Can you work these out from the model? Positions are in its coordinate system, mm. A direction names the side the tool comes from. Coordinates: 2 decimals unless noted, no trailing zeros. Write each loop counter-clockwise with the first axis right and the second up, starting at its lowest first coordinate (ties: lowest second). Pieces come first, ordered by that corner, then holes. Notation, with made-up numbers: (51, 58.25) -> (102, 58.25) arc R18 cw to (102, 84.25) -> close; hole circle Ø4 at (9, 0). An arc over 180 degrees is marked (long way). Use one line per item in the form item = value.
Autodesk Inventor part; units mm, degrees
ref_plane "Work Plane1" through (0, 20, -19.05) normal (-1, 0, 0) x (0, 0, 1)
ref_plane "Work Plane2" through (6.5, 7, 0) normal (0, 0, -1) x (-1, 0, 0)
ref_plane "YZ Plane" through (0, 0, 0) normal (1, 0, 0) x (0, 1, 0)
sketch "Sketch1" plane through (0, 0, 0) normal (0, 1, 0) x (-1, 0, 0)
  line L0 (17.5, 19.05) -> (-17.5, 19.05)
  line L1 (-17.5, 19.05) -> (-17.5, -19.05)
  line L2 (-17.5, -19.05) -> (17.5, -19.05)
  line L3 (17.5, -19.05) -> (17.5, 19.05)
  line L4 (17.5, 19.05) -> (-17.5, -19.05) construction
  line L5 (-17.5, 19.05) -> (17.5, -19.05) construction
  point P0 (0, 0)
  dimension "d0" = 38.1
  dimension "d1" = 35
extrude "Extrusion1" add sketch "Sketch1" along normal blind 20
shell "Shell1" thickness 2 removed faces 1 at (5.8333, 20, -6.35)
sketch "Sketch2" plane through (-15.5, 2, 17.05) normal (0, 1, 0) x (1, 0, 0)
  line L0 (31, 34.1) -> (0, 34.1)
  line L1 (31, 0) -> (31, 34.1)
  line L2 (0, 34.1) -> (31, 34.1)
  line L3 (31, 34.1) -> (31, 0)
  line L4 (31, 0) -> (0, 0)
  line L5 (0, 0) -> (0, 34.1)
  point P0 (15.5, 17.05)
extrude "Extrusion2" add sketch "Sketch2" along normal blind 15.5
sketch "Sketch3" plane through (0, 20, 0) normal (0, 1, 0) x (1, 0, 0)
  line L0 (17.5, 19.05) -> (-17.5, 19.05)
  line L1 (-17.5, -19.05) -> (17.5, -19.05)
  line L2 (0, 19.05) -> (-6.5, 19.05)
  line L3 (-6.5, 19.05) -> (-6.5, -19.05)
  line L4 (-6.5, -19.05) -> (0, -19.05)
  line L5 (0, -19.05) -> (0, 19.05)
  point P0 (0, 0)
  dimension "d7" = 6.5
extrude "Extrusion3" cut sketch "Sketch3" against normal blind 13
ref_plane "Work Plane1" through (0, 20, -19.05) normal (-1, 0, 0) x (0, 0, 1)
mirror "Mirror1" about plane through (0, 20, -19.05) normal (-1, 0, 0) of "Extrusion3"
sketch "Sketch4" plane through (-15.5, 17.5, 17.05) normal (0, 1, 0) x (1, 0, 0)
  line L0 (22, -2) -> (22, 36.1)
  line L1 (22, 17.05) -> (26, 17.05)
  line L2 (26, 17.05) -> (26, 29.55)
  line L3 (26, 29.55) -> (22, 29.55)
  line L4 (22, 29.55) -> (22, 17.05)
  point P0 (15.5, 17.05)
  dimension "d11" = 4
  dimension "d12" = 12.5
extrude "Extrusion4" cut sketch "Sketch4" against normal up to surface (10.5 mm away)
sketch "Sketch5" plane through (-15.5, 17.5, 17.05) normal (0, 1, 0) x (1, 0, 0)
  line L0 (26, 17.05) -> (26, 29.55)
  line L1 (26, 17.05) -> (28.5, 17.05)
  line L2 (28.5, 17.05) -> (28.5, 26.85)
  line L3 (28.5, 26.85) -> (26, 26.85)
  line L4 (26, 26.85) -> (26, 17.05)
  point P0 (15.5, 17.05)
  dimension "d15" = 9.8
  dimension "d16" = 2.5
extrude "Extrusion5" cut sketch "Sketch5" against normal blind 12.7
sketch "Sketch6" plane through (0, 20, 0) normal (0, 1, 0) x (1, 0, 0)
  line L0 (15.5, 17.05) -> (15.5, -17.05)
  line L1 (15.5, 0) -> (19.9746, 0)
  line L2 (19.9746, 0) -> (19.9746, 7.5)
  line L3 (19.9746, 7.5) -> (15.5, 7.5)
  line L4 (15.5, 7.5) -> (15.5, 0)
  point P0 (0, 0)
  dimension "d19" = 7.5
extrude "Extrusion6" cut sketch "Sketch6" against normal up to surface (2.5 mm away)
ref_plane "Work Plane2" through (6.5, 7, 0) normal (0, 0, -1) x (-1, 0, 0)
mirror "Mirror2" about plane through (6.5, 7, 0) normal (0, 0, -1) of "Extrusion4", "Extrusion5", "Extrusion6"
sketch "Sketch7" plane through (-17.5, 0, -19.05) normal (-1, 0, 0) x (0, 0, 1)
  circle A0 centre (19.05, 12.14) radius 2.6
  line L0 (0, 20) -> (38.1, 20)
  point P0 (19.05, 0)
  dimension "d23" = 5.2
  dimension "d24" = 7.86
extrude "Extrusion7" cut sketch "Sketch7" against normal up to surface (11 mm away)
sketch "Sketch8" plane through (-17.5, 0, -19.05) normal (-1, 0, 0) x (0, 0, 1)
  circle A0 centre (19.05, 12.14) radius 2.6
  circle A1 centre (19.05, 12.14) radius 3.2
  point P0 (19.05, 0)
  dimension "d27" = 6.4
extrude "Extrusion8" cut sketch "Sketch8" against normal blind 9.5
fillet "Fillet1" radius 2 8 edges at (15.5, 18.75, -17.05) (-15.5, 18.75, -17.05) (-15.5, 18.75, 17.05) (15.5, 18.75, 17.05) (-17.5, 10, 19.05) (17.5, 10, 19.05) (17.5, 10, -19.05) (-17.5, 10, -19.05)
properties part number "Enclosure_Bottom V1D6"
Q1. Suppose I cut it at D-D (y = 12.14). Write out the boundary of the cut face in (x, z), then the cut area to 3 significant figures.
Return value:
outline = (-17.5, -17.05) arc R2 ccw to (-15.5, -19.05) -> (-6.5, -19.05) -> (-6.5, -2.6) -> (-8, -2.6) -> (-8, -3.2) -> (-17.5, -3.2) -> close; (-17.5, 3.2) -> (-8, 3.2) -> (-8, 2.6) -> (-6.5, 2.6) -> (-6.5, 19.05) -> (-15.5, 19.05) arc R2 ccw to (-17.5, 17.05) -> close; (6.5, -19.05) -> (15.5, -19.05) arc R2 ccw to (17.5, -17.05) -> (17.5, 17.05) arc R2 ccw to (15.5, 19.05) -> (6.5, 19.05) -> (6.5, 12.5) -> (10.5, 12.5) -> (10.5, 9.8) -> (13, 9.8) -> (13, -9.8) -> (10.5, -9.8) -> (10.5, -12.5) -> (6.5, -12.5) -> close
area = 617 mm2
Q2. Suppose I cut it at C-C (x = 12.5). Write out the boundary of the cut face in (y, z).
Return value:
outline = (0, -19.05) -> (20, -19.05) -> (20, -17.05) -> (17.5, -17.05) -> (17.5, -9.8) -> (4.8, -9.8) -> (4.8, 9.8) -> (17.5, 9.8) -> (17.5, 17.05) -> (20, 17.05) -> (20, 19.05) -> (0, 19.05) -> close
Q3. For faces 4 (the cylindrical face through (14.9, 18.73, -16.48)), 5 (the flat face through (6.5, 12, -16)), 6 (the flat face through (16, 20, 15)), which set-ups out of +Z, -Z, +X, -X, +Y, -Y let a thin tool reach every point of the face, with its end or its side?
Return value:
face_4 = +Y
face_5 = +Z, -Z, +Y
face_6 = +Z, -Z, +X, -X, +Y
Q4. If I drill on line 1 (Y direction, x = -10, z = 0); line 2 (X direction, y = 15, z = -15); line 3 (X direction, y = 16.5, z = -3.5), over which ranges is the centre line in solid material (lowest first)? Write a range as from..to.
Return value:
line_1 = 0..8.94, 15.34..17.5
line_2 = -17.5..-6.5, 6.5..17.5
line_3 = -17.5..-6.5, 13..17.5
Q5. Suppose I cut it at B-B (z = 0). Write out the boundary of the cut face in (x, y).
Return value:
outline = (-17.5, 0) -> (17.5, 0) -> (17.5, 17.5) -> (13, 17.5) -> (13, 4.8) -> (10.5, 4.8) -> (10.5, 7) -> (-6.5, 7) -> (-6.5, 9.54) -> (-8, 9.54) -> (-8, 8.94) -> (-17.5, 8.94) -> close; (-17.5, 15.34) -> (-8, 15.34) -> (-8, 14.74) -> (-6.5, 14.74) -> (-6.5, 17.5) -> (-15.5, 17.5) -> (-15.5, 20) -> (-17.5, 20) -> close
Q6. Will these pins go through, and if not, where does the flat tip stop? pin 1 (3 mm diameter, centred on x = 12, z = -4, fed in from +Y); pin 2 (3 mm diameter, centred on y = 19, z = -6.5, fed in from +X); pin 3 (4 mm diameter, centred on y = 12.14, z = 0, fed in from -X); pin 4 (3.5 mm diameter, centred on x = 11, z = 3, fed in from +Y).
Return value:
pin_1 = 17.5
pin_2 = 17.5
pin_3 = 13
pin_4 = 7
Q7. Suppose I cut it at A-A (y = 17). Write out the boundary of the cut face in (x, z), then the cut area to 3 significant figures.
Return value:
outline = (-17.5, -17.05) arc R2 ccw to (-15.5, -19.05) -> (-6.5, -19.05) -> (-6.5, 19.05) -> (-15.5, 19.05) arc R2 ccw to (-17.5, 17.05) -> close; (6.5, -19.05) -> (15.5, -19.05) arc R2 ccw to (17.5, -17.05) -> (17.5, 17.05) arc R2 ccw to (15.5, 19.05) -> (6.5, 19.05) -> (6.5, 12.5) -> (10.5, 12.5) -> (10.5, 9.8) -> (13, 9.8) -> (13, -9.8) -> (10.5, -9.8) -> (10.5, -12.5) -> (6.5, -12.5) -> close
area = 686 mm2
Q8. Thinking about a two-plate mould opening in Z: for faces 1 (the flat face through (-15.5, 19, 0)), 2 (the cylindrical face through (-16.93, 10.14, 18.45)), 3 (the flat face through (16, 20, -15)), which applies, released by +Z, released by -Z, zero draft, split by the parting line, or undercut?
Return value:
face_1 = undercut
face_2 = released by +Z
face_3 = zero draft
